from build123d import *

# Parameters (mm, degrees)
SKETCH1_W                    = 177.8
SKETCH1_H                    = 152.4
BASE_FLANGE1_DEPTH           = 2.05232
EDGE_FLANGE1_STRIP_W         = 9.68248
EDGE_FLANGE1_STRIP_H         = 2.05232
EDGE_FLANGE1_STRIP_CUT_DEPTH = 177.8
EDGE_FLANGE1_DEPTH           = 177.8
SKETCH9_R                    = 2.032
CUT_EXTRUDE1_DEPTH           = 2.54
SKETCH10_R                   = 14.2875
CUT_EXTRUDE2_DEPTH           = 2.54


# Sheet-metal steps are written as plain solids
with BuildPart() as part:
    # Sketch1 → Base-Flange1 (new body)
    with BuildSketch(Plane(origin=(0, 0, 0), x_dir=(1, 0, 0), z_dir=(0, 1, 0))):
        with Locations((-5549.9, 2677.885714286)):
            Rectangle(SKETCH1_W, SKETCH1_H)
    extrude(amount=-BASE_FLANGE1_DEPTH)

    # Edge-Flange1 strip (across the edge) → Edge-Flange1 strip cut (cut)
    with BuildSketch(Plane(origin=(-5638.8, 0, -2601.685714286), x_dir=(0, 0, -1), z_dir=(1, 0, 0))):
        with Locations((-2.05232, -1.02616)):
            Rectangle(EDGE_FLANGE1_STRIP_W, EDGE_FLANGE1_STRIP_H)
    extrude(amount=EDGE_FLANGE1_STRIP_CUT_DEPTH, mode=Mode.SUBTRACT)

    # Edge-Flange1 section (across the edge) → Edge-Flange1 (add)
    with BuildSketch(Plane(origin=(-5638.8, 0, -2601.685714286), x_dir=(0, 0, -1), z_dir=(1, 0, 0))):
        with BuildLine():
            Line((0, 0.7366), (0, 16.99768))
            Line((0, 16.99768), (2.05232, 16.99768))
            Line((2.05232, 16.99768), (2.05232, 0.7366))
            ThreePointArc((2.05232, 0.7366), (2.268065145, 0.215745145), (2.78892, 0))
            Line((2.78892, 0), (2.78892, -2.05232))
            ThreePointArc((2.78892, -2.05232), (0.816855756, -1.235464244), (0, 0.7366))
        make_face()
    extrude(amount=EDGE_FLANGE1_DEPTH)

    # Sketch9 → Cut-Extrude1 (cut)
    with BuildSketch(Plane(origin=(0, 0, -2603.738034286), x_dir=(-1, 0, 0), z_dir=(0, 0, -1))):
        with Locations((5626.1, 6.83768)):
            Circle(SKETCH9_R)
        with Locations((5600.7, 6.83768)):
            Circle(SKETCH9_R)
        with Locations((5575.3, 6.83768)):
            Circle(SKETCH9_R)
        with Locations((5549.9, 6.83768)):
            Circle(SKETCH9_R)
        with Locations((5524.5, 6.83768)):
            Circle(SKETCH9_R)
        with Locations((5499.1, 6.83768)):
            Circle(SKETCH9_R)
        with Locations((5473.7, 6.83768)):
            Circle(SKETCH9_R)
    extrude(amount=-CUT_EXTRUDE1_DEPTH, mode=Mode.SUBTRACT)

    # Sketch10 → Cut-Extrude2 (cut)
    with BuildSketch(Plane.XZ.offset(2.05232)):
        with Locations(Location((-5549.9, -2637.733394286, 0), (0, 0, 270))):
            Circle(SKETCH10_R)
    extrude(amount=-CUT_EXTRUDE2_DEPTH, mode=Mode.SUBTRACT)


solid = part.part
The listing builds one solid part. Answer for the finished solid, in the listing's coordinates (mm). A direction names the side the tool comes from. Coordinates: 2 decimals unless noted, no trailing zeros. Write each loop counter-clockwise with the first axis right and the second up, starting at its lowest first coordinate (ties: lowest second). Pieces come first, ordered by that corner, then holes. Notation, with made-up numbers: (-24, 82.5) - (-8, 82.5) arc R12 ccw to (-8, 91.5) - close; hole circle Ø1 at (25.5, -7.75). An arc over 180 degrees is marked (long way). Return JSON: item names as keys, results as strings.
1. The part is cut by section B-B on x = -5473.7. Determine the outline of the cut face in (y, z), then the cut area to 3 significant figures.
Final values:
{"outline": "(-2.05, -2754.09) - (0, -2754.09) - (0, -2604.47) arc R0.74 cw to (0.74, -2603.74) - (4.81, -2603.74) - (4.81, -2601.69) - (0.74, -2601.69) arc R2.79 ccw to (-2.05, -2604.47) - close; (8.87, -2603.74) - (17, -2603.74) - (17, -2601.69) - (8.87, -2601.69) - close", "area": "338 mm^2"}
2. Each of these flat-tipped pins is pushed along its axis until it touches: pin 1 Ø5.5 at (x, y) = (-5600.7, 6.84) entering from -Z; pin 2 Ø4.5 at (x, y) = (-5473.7, 6.84) entering from +Z; pin 3 Ø4 at (x, z) = (-5531.5, -2631) entering from +Y. Where does it stop, or does it pass through?
Final values:
{"pin 1": "z = -2603.74", "pin 2": "z = -2601.69", "pin 3": "y = 0"}
3. Consider line 1 along Y through (x, z) = (-5626.1, -2602.3); line 2 along Z through (x, y) = (-5551.5, 4.5); line 3 along Z through (x, y) = (-5549.9, -0.55). Determine where each line is inside the solid, lowest interval first.
Final values:
{"line 1": "-1.01 to 4.81, 8.87 to 17", "line 2": "-2603.74 to -2601.69", "line 3": "-2754.09 to -2652.02, -2623.45 to -2602"}
4. Which of the six approach directions +Z, -Z, +X, -X, +Y, -Y give full straight-line access (tool end or side, diameter ignored) to faces 1 (the face through (-5551, 9, -2603.738)), 2 (the face through (-5638.8, -1, -2678))?
Final values:
{"face 1": "-Z, +X, -X, +Y", "face 2": "+Z, -Z, -X, +Y, -Y"}
5. The part is cut by section D-D on x = -5507.5. Determine the outline of the cut face in (y, z).
Final values:
{"outline": "(-2.05, -2754.09) - (0, -2754.09) - (0, -2604.47) arc R0.74 cw to (0.74, -2603.74) - (17, -2603.74) - (17, -2601.69) - (0.74, -2601.69) arc R2.79 ccw to (-2.05, -2604.47) - close"}
6. The part is cut by section A-A on x = -5549.9. Determine the outline of the cut face in (y, z).
Final values:
{"outline": "(-2.05, -2754.09) - (0, -2754.09) - (0, -2652.02) - (-2.05, -2652.02) - close; (-2.05, -2623.45) - (0, -2623.45) - (0, -2604.47) arc R0.74 cw to (0.74, -2603.74) - (4.81, -2603.74) - (4.81, -2601.69) - (0.74, -2601.69) arc R2.79 ccw to (-2.05, -2604.47) - close; (8.87, -2603.74) - (17, -2603.74) - (17, -2601.69) - (8.87, -2601.69) - close"}
7. The part is cut by section C-C on z = -2654.5. Determine the outline of the cut face in (x, y).
Final values:
{"outline": "(-5638.8, -2.05) - (-5461, -2.05) - (-5461, 0) - (-5638.8, 0) - close"}
8. For a pull along Z with two mould halves and no side action, classify faces 3 (the face through (-5563.85, -1.04, -2634.64)), 4 (the face through (-5461, -1, -2678)), 5 (the face through (-5551, 9, -2601.686)) as +Z half, -Z half, draft (parallel to the pull), parting line (faces both ways), or undercut.
Final values:
{"face 3": "undercut", "face 4": "draft", "face 5": "+Z half"}
